```python
from build123d import *

# Parameters (mm, degrees)
SKETCH_1_W          = 30
SKETCH_1_H          = 12
EXTRUDE_1_DEPTH     = 6
CUT_EXTRUDE_2_REACH = 22.125
SKETCH_4_R          = 1.65


with BuildPart() as part:
    # 草图1 → 凸台-拉伸1 (new body)
    with BuildSketch(Plane(origin=(0, 0, 0), x_dir=(1, 0, 0), z_dir=(0, 1, 0))):
        with Locations((0, 6)):
            Rectangle(SKETCH_1_W, SKETCH_1_H)
    extrude(amount=EXTRUDE_1_DEPTH)

    # 草图2 → 切除-旋转1 (revolve, cut)
    with BuildSketch(Plane.XY):
        Polygon((-8, 0), (0, 0), (0, 3), (-9, 3), (-9, 1), (-8, 1), align=None)
        Polygon((-9, 3), (0, 3), (0, 6), (-8, 6), (-8, 5), (-9, 5), align=None)
    revolve(axis=Axis((0, 0, 0), (0, 1, 0)), mode=Mode.SUBTRACT)

    # 草图4 → 切除-拉伸2 (cut, up to next)
    with BuildSketch(Plane(origin=(0, 0, -12), x_dir=(-1, 0, 0), z_dir=(0, 0, -1)), mode=Mode.PRIVATE) as cut_extrude_2_sk1:
        with Locations((-12, 3)):
            Circle(SKETCH_4_R)
    cut_extrude_2_tool1 = extrude(cut_extrude_2_sk1.sketch, amount=-CUT_EXTRUDE_2_REACH, mode=Mode.PRIVATE) & part.part
    cut_extrude_2 = cut_extrude_2_tool1.solids().sort_by_distance((12, 3, -12))[0]
    add(cut_extrude_2, mode=Mode.SUBTRACT)

    # 镜向1: 切除-拉伸2 across plane
    add(cut_extrude_2.mirror(Plane(origin=(0, 0, 0), x_dir=(0, 0, 1), z_dir=(1, 0, 0))), mode=Mode.SUBTRACT)


solid = part.part
```
Design review of the part built by this model. Coordinates are the model's own, in mm. A direction names the side the tool comes from. Give positions to 0.01 mm unless a question says otherwise; leave off trailing zeros. Order: outer loops, then holes, each group sorted by start corner. A loop starts at its lowest first (then second) coordinate and runs counter-clockwise, first axis right, second up. Notation, with made-up numbers: (-18, -8.75) - (-5, -8.75) arc R26 ccw to (-5, 14.25) - close; hole circle Ø11 at (29.5, 33). An arc over 180 degrees is marked (long way). Use a Markdown table: item, result. Add a question column.
(1) Machinability: for faces 4 (the face through (10.7, 1.6, 0)), 5 (the face through (0, 3, -9)), which of the approach directions +Z, -Z, +X, -X, +Y, -Y give a long, thin tool a straight path to every point of the face, cutting with its end or side? Answer none if there is none.
(2) Add section A-A on y = 3. Give the boundary of the cut face in (x, z).
(3) Clearance check with flat-ended pins moving along their axes: P1, Ø2, axis at x = -4.5, y = 1, coming from the +Z side; P2, Ø3, axis at x = -12, y = 3, coming from the +Z side. State where each tip first meets the part, or that it passes through.
(4) Wall thickness on probe 1 along Y at (x, z) = (-12, -9); probe 2 along X at (y, z) = (2.4, -10); probe 3 along X at (y, z) = (3.8, -8): over which ranges is each line inside the solid? List them lowest first. Write a range as [from, to].
(5) Mouldability with a two-part tool opening along X and no side actions: class faces 1 (the face through (0.04, 1, -8.15)), 2 (the face through (-15, 3, -6)), 3 (the face through (0, 0, -9)) as +X half, -X half, draft (parallel to the pull), parting line (faces both ways), or undercut.
(6) Add section C-C on z = -2.5. Give the boundary of the cut face in (x, y).
(7) Add section D-D on x = 0. Give the boundary of the cut face in (y, z), then the cut area to 3 significant figures.
(8) Add section B-B on x = -12. Give the boundary of the cut face in (y, z).
Report:
| question | item | result |
|---|---|---|
| 1 | face 4 | +Z, +X, -X, +Y, -Y |
| 1 | face 5 | +Z |
| 2 | outline | (-15, -12) - (-13.65, -12) - (-13.65, 0) - (-15, 0) - close; (-10.35, -12) - (10.35, -12) - (10.35, 0) - (9, 0) arc R9 cw to (-9, 0) - (-10.35, 0) - close; (13.65, -12) - (15, -12) - (15, 0) - (13.65, 0) - close |
| 3 | P1 | stops at z = -5.81 |
| 3 | P2 | passes through |
| 4 | probe 1 | y = [0, 1.35], [4.65, 6] |
| 4 | probe 2 | x = [-15, -13.54], [-10.46, 10.46], [13.54, 15] |
| 4 | probe 3 | x = [-15, -13.44], [-10.56, -4.12], [4.12, 10.56], [13.44, 15] |
| 5 | face 1 | undercut |
| 5 | face 2 | -X half |
| 5 | face 3 | draft |
| 6 | outline | (-15, 0) - (-7.6, 0) - (-7.6, 1) - (-8.65, 1) - (-8.65, 5) - (-7.6, 5) - (-7.6, 6) - (-15, 6) - close; (7.6, 0) - (15, 0) - (15, 6) - (7.6, 6) - (7.6, 5) - (8.65, 5) - (8.65, 1) - (7.6, 1) - close; hole circle Ø3.3 at (-12, 3); hole circle Ø3.3 at (12, 3) |
| 7 | outline | (0, -12) - (6, -12) - (6, -8) - (5, -8) - (5, -9) - (1, -9) - (1, -8) - (0, -8) - close |
| 7 | area | 20.0 mm² |
| 8 | outline | (0, -12) - (1.35, -12) - (1.35, 0) - (0, 0) - close; (4.65, -12) - (6, -12) - (6, 0) - (4.65, 0) - close |
